Source: CAD feature listing. Evaluate the final solid. Frame: model axes, mm. Round coordinates to 2 decimals unless told otherwise and drop trailing zeros. Loops run counter-clockwise (first coordinate to the right, second up) from the corner with the lowest first, then second, coordinate; pieces in that order, holes last.
(1) First-contact query: pin 1 Ø3 at (x, y) = (6.35, 75) entering from +Z. Flat tip, straight axial feed; report the tip coordinate or a pass-through.
(2) Material intervals for probe 1 along Y at (x, z) = (6.5, 6.75); probe 2 along Z at (x, y) = (8.75, 42.5); probe 3 along Y at (x, z) = (7.75, 8), sorted ascending.
(3) Section B-B, the plane x = 5.5. Return the cut outline in (y, z).
(4) Section C-C, the plane z = 6.75. Return the cut outline in (x, y).
(5) Mould query, pull axis Z, two halves, no side actions, for faces 1 (the flat face through (6, 39, 0)), 2 (the cylindrical face through (6.439, 47.498, 6.203)), 3 (the flat face through (6, 39, 12.7)), 4 (the cylindrical face through (6.61, 76.983, 6.261)). Classes: pulls with the +Z half, pulls with the -Z half, needs draft (parallel to the pull), parting line crosses it, or undercut.
(6) Section D-D, the plane z = 9.75. Return the cut outline in (x, y), plus the area to 3 significant figures.
(7) Section A-A, the plane y = 15. Return the cut outline in (x, z).
```python
from build123d import *

# Parameters (mm, degrees)
SKETCH1_W           = 12.7
SKETCH1_H           = 12.7
BOSS_EXTRUDE1_DEPTH = 80
CUT_EXTRUDE1_DEPTH  = 80
SKETCH3_R           = 2
CUT_EXTRUDE2_DEPTH  = 80


with BuildPart() as part:
    # Sketch1 → Boss-Extrude1 (new body)
    with BuildSketch(Plane(origin=(0, 0, 0), x_dir=(1, 0, 0), z_dir=(0, 1, 0))):
        with Locations((6.35, -6.35)):
            Rectangle(SKETCH1_W, SKETCH1_H)
    extrude(amount=BOSS_EXTRUDE1_DEPTH)

    # Sketch2 → Cut-Extrude1 (cut)
    with BuildSketch(Plane(origin=(12.7, 0, 0), x_dir=(0, 0, -1), z_dir=(1, 0, 0))):
        with BuildLine():
            ThreePointArc((-10.680127019, 40), (-6.35, 32.5), (-2.019872981, 40))
            ThreePointArc((-2.019872981, 40), (-6.35, 47.5), (-10.680127019, 40))
        make_face()
    extrude(amount=-CUT_EXTRUDE1_DEPTH, mode=Mode.SUBTRACT)

    # Sketch3 → Cut-Extrude2 (cut)
    with BuildSketch(Plane(origin=(0, 0, 0), x_dir=(-1, 0, 0), z_dir=(0, 0, -1))):
        with Locations((-6.35, 5)):
            Circle(SKETCH3_R)
        with Locations((-6.35, 15)):
            Circle(SKETCH3_R)
        with Locations((-6.35, 75)):
            Circle(SKETCH3_R)
        with Locations((-6.35, 65)):
            Circle(SKETCH3_R)
    extrude(amount=-CUT_EXTRUDE2_DEPTH, mode=Mode.SUBTRACT)


solid = part.part
```
Output values:
1. pin 1: passes through
2. probe 1: y = 0 to 3.01, 6.99 to 13.01, 16.99 to 32.52, 47.48 to 63.01, 66.99 to 73.01, 76.99 to 80
2. probe 2: z = 0 to 1.35, 11.35 to 12.7
2. probe 3: y = 0 to 3.57, 6.43 to 13.57, 16.43 to 32.78, 47.22 to 63.57, 66.43 to 73.57, 76.43 to 80
3. outline: (0, 0) - (3.19, 0) - (3.19, 12.7) - (0, 12.7) - close; (6.81, 0) - (13.19, 0) - (13.19, 12.7) - (6.81, 12.7) - close; (16.81, 0) - (63.19, 0) - (63.19, 12.7) - (16.81, 12.7) - close; (66.81, 0) - (73.19, 0) - (73.19, 12.7) - (66.81, 12.7) - close; (76.81, 0) - (80, 0) - (80, 12.7) - (76.81, 12.7) - close; hole (40, 2.02) arc R5 ccw (long way) to (40, 10.68) arc R5 ccw (long way) to start
4. outline: (0, 0) - (12.7, 0) - (12.7, 32.52) - (0, 32.52) - close; (0, 47.48) - (12.7, 47.48) - (12.7, 80) - (0, 80) - close; hole circle Ø4 at (6.35, 5); hole circle Ø4 at (6.35, 15); hole circle Ø4 at (6.35, 65); hole circle Ø4 at (6.35, 75)
5. face 1: pulls with the -Z half
5. face 2: undercut
5. face 3: pulls with the +Z half
5. face 4: needs draft
6. outline: (0, 0) - (12.7, 0) - (12.7, 33.83) - (0, 33.83) - close; (0, 46.17) - (12.7, 46.17) - (12.7, 80) - (0, 80) - close; hole circle Ø4 at (6.35, 5); hole circle Ø4 at (6.35, 15); hole circle Ø4 at (6.35, 65); hole circle Ø4 at (6.35, 75)
6. area: 809 mm2
7. outline: (0, 0) - (4.35, 0) - (4.35, 12.7) - (0, 12.7) - close; (8.35, 0) - (12.7, 0) - (12.7, 12.7) - (8.35, 12.7) - close
